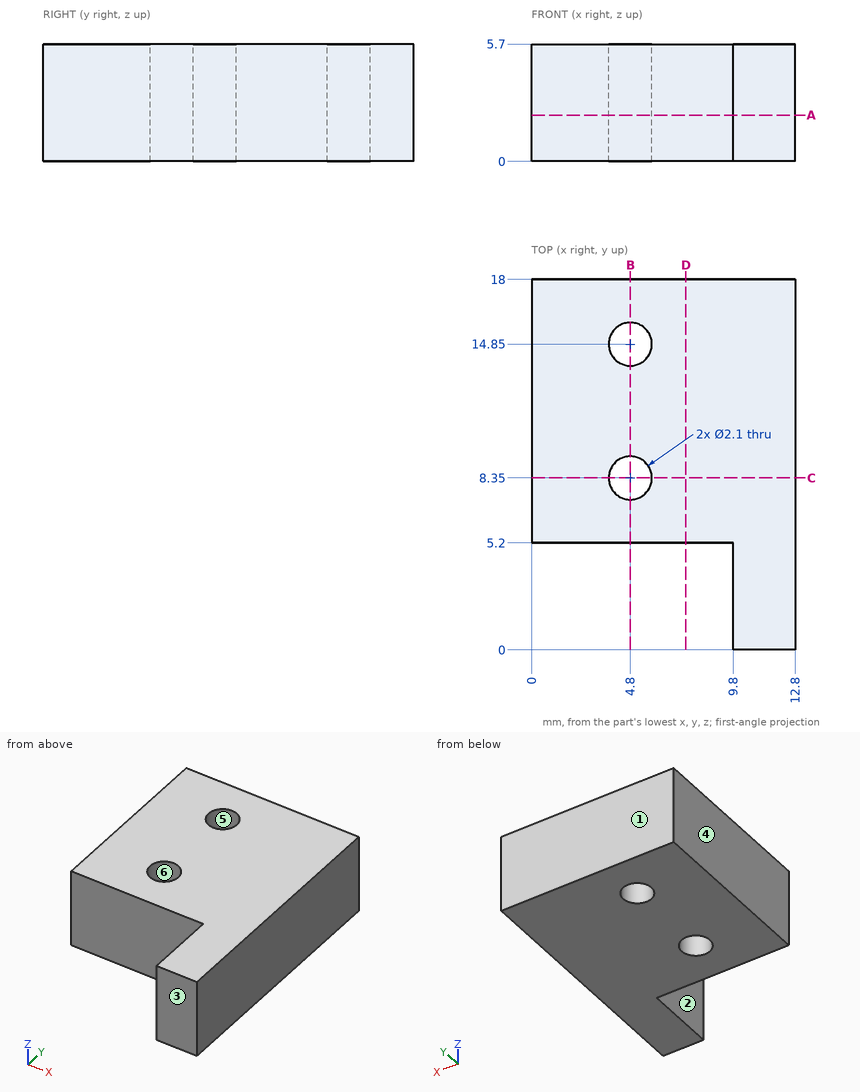
Part print with two shaded views. Sizes in mm from the minimum x, y, z corner. A direction names the side the tool comes from. Give positions to 0.01 mm unless a question says otherwise; leave off trailing zeros. Order: outer loops, then holes, each group sorted by start corner. A loop starts at its lowest first (then second) coordinate and runs counter-clockwise, first axis right, second up.
1) Wall check: probe 1 along Y at (x, z) = (5, 2.4); probe 2 along X at (y, z) = (14.85, 3.85); probe 3 along Y at (x, z) = (9, 4.05). Give the ranges that are in metal, low to high.
2) Mould opens along Y. For the marked faces 3, 4, 5 and 6 say: +Y half, -Y half, draft (parallel to the pull), parting line (faces both ways), or undercut.
3) Pin check, flat tip, straight feed: pin 1 (1.7 mm diameter, centred on x = 7, z = 3.5, fed in from -Y). Stop position of the tip, or through.
4) Saw through at B-B, the plane x = 4.8. Write the cut outline in (y, z), then the cut area to 3 significant figures.
5) Saw through at D-D, the plane x = 7.5. Write the cut outline in (y, z), then the cut area to 3 significant figures.
6) Saw through at C-C, the plane y = 8.35. Write the cut outline in (x, z), then the cut area to 3 significant figures.
7) 3-axis set-ups, long thin cutter, end or side, ignore diameter. For the marked faces 1 and 2: which of +Z, -Z, +X, -X, +Y, -Y reach the whole face in a straight line?
8) Saw through at A-A, the plane z = 2.25. Write the cut outline in (x, y), then the cut area to 3 significant figures.
Computed:
1. probe 1: y = 5.2 to 7.32, 9.38 to 13.82, 15.88 to 18
1. probe 2: x = 0 to 3.75, 5.85 to 12.8
1. probe 3: y = 5.2 to 18
2. face 3: -Y half
2. face 4: draft
2. face 5: undercut
2. face 6: undercut
3. pin 1: stops at y = 5.2
4. outline: (5.2, 0) - (7.3, 0) - (7.3, 5.7) - (5.2, 5.7) - close; (9.4, 0) - (13.8, 0) - (13.8, 5.7) - (9.4, 5.7) - close; (15.9, 0) - (18, 0) - (18, 5.7) - (15.9, 5.7) - close
4. area: 49.0 mm2
5. outline: (5.2, 0) - (18, 0) - (18, 5.7) - (5.2, 5.7) - close
5. area: 73.0 mm2
6. outline: (0, 0) - (3.75, 0) - (3.75, 5.7) - (0, 5.7) - close; (5.85, 0) - (12.8, 0) - (12.8, 5.7) - (5.85, 5.7) - close
6. area: 61.0 mm2
7. face 1: +Z, -Z, +X, -X, +Y
7. face 2: +Z, -Z, -X, -Y
8. outline: (0, 5.2) - (9.8, 5.2) - (9.8, 0) - (12.8, 0) - (12.8, 18) - (0, 18) - close; hole circle Ø2.1 at (4.8, 8.35); hole circle Ø2.1 at (4.8, 14.85)
8. area: 173 mm2
